```python
from build123d import *

# Parameters (mm, degrees)
BOSS_EXTRUDE1_DEPTH = 22.34
SKETCH3_W           = 42.42
SKETCH3_H           = 6
CUT_EXTRUDE1_DEPTH  = 20.34
SKETCH4_W           = 45.42
SKETCH4_H           = 3.5
CUT_EXTRUDE2_DEPTH  = 20.34
SKETCH6_R           = 0.6
SKETCH6_R_2         = 0.45
SKETCH6_R_3         = 2.25
BOSS_EXTRUDE2_DEPTH = 4
BOSS_EXTRUDE3_START = 2
SKETCH7_R           = 2.25
SKETCH7_R_2         = 1.9
BOSS_EXTRUDE3_DEPTH = 0.5
SKETCH8_W           = 42.42
SKETCH8_H           = 1.5
BOSS_EXTRUDE4_DEPTH = 2
BOSS_EXTRUDE5_DEPTH = 1
FILLET1_R           = 0.5


with BuildPart() as part:
    # Sketch1 → Boss-Extrude1 (new body)
    with BuildSketch(Plane(origin=(0, 0, 0), x_dir=(1, 0, 0), z_dir=(0, 1, 0))):
        Polygon((47.42, 0), (47.42, 6), (45.42, 6), (0, 6), (-2, 6), (-2, 0), (0, 0), (45.42, 0), align=None)
    extrude(amount=BOSS_EXTRUDE1_DEPTH)

    # Sketch3 → Cut-Extrude1 (cut)
    with BuildSketch(Plane(origin=(0, 22.34, 0), x_dir=(1, 0, 0), z_dir=(0, 1, 0))):
        with Locations((22.71, 3)):
            Rectangle(SKETCH3_W, SKETCH3_H)
    extrude(amount=-CUT_EXTRUDE1_DEPTH, mode=Mode.SUBTRACT)

    # Sketch4 → Cut-Extrude2 (cut)
    with BuildSketch(Plane(origin=(0, 22.34, 0), x_dir=(1, 0, 0), z_dir=(0, 1, 0))):
        with Locations((22.71, 2.75)):
            Rectangle(SKETCH4_W, SKETCH4_H)
    extrude(amount=-CUT_EXTRUDE2_DEPTH, mode=Mode.SUBTRACT)

    # Sketch6 → Boss-Extrude2 (add)
    with BuildSketch(Plane.XZ):
        with BuildLine():
            Line((12.71, -6), (19.146099522, -16))
            Line((19.146099522, -16), (19.146099522, -36))
            ThreePointArc((19.146099522, -36), (22.71, -39.563900478), (26.273900478, -36))
            Line((26.273900478, -36), (26.273900478, -16))
            Line((26.273900478, -16), (32.71, -6))
            Line((32.71, -6), (12.71, -6))
        make_face()
        with Locations((22.71, -16)):
            Circle(SKETCH6_R, mode=Mode.SUBTRACT)
        with Locations((22.71, -24.75)):
            Circle(SKETCH6_R_2, mode=Mode.SUBTRACT)
        with Locations((22.71, -32.75)):
            Circle(SKETCH6_R_3, mode=Mode.SUBTRACT)
    extrude(amount=-BOSS_EXTRUDE2_DEPTH)

    # Sketch7 → Boss-Extrude3 (add)
    with BuildSketch(Plane(origin=(0, 2, 0), x_dir=(1, 0, 0), z_dir=(0, 1, 0)).offset(BOSS_EXTRUDE3_START)):
        with Locations((22.71, 32.75)):
            Circle(SKETCH7_R)
        with Locations((22.71, 32.75)):
            Circle(SKETCH7_R_2, mode=Mode.SUBTRACT)
    extrude(amount=-BOSS_EXTRUDE3_DEPTH)

    # Sketch8 → Boss-Extrude4 (add)
    with BuildSketch(Plane(origin=(0, 2, 0), x_dir=(1, 0, 0), z_dir=(0, 1, 0))):
        with Locations((22.71, 5.25)):
            Rectangle(SKETCH8_W, SKETCH8_H)
    extrude(amount=BOSS_EXTRUDE4_DEPTH)

    # Sketch11 → Boss-Extrude5 (add)
    with BuildSketch(Plane.XY):
        Polygon((1.5, 4), (3.5, 2), (1.5, 2), align=None)
        Polygon((43.92, 4), (41.92, 2), (43.92, 2), align=None)
    extrude(amount=-BOSS_EXTRUDE5_DEPTH)

    # Fillet1
    fillet1_edges = [part.edges().sort_by_distance(p)[0] for p in [
        (1.5, 4, -5.25),
        (43.92, 4, -5.25),
        (47.42, 22.34, -3),
        (-2, 22.34, -3),
        (1.5, 22.34, -5.25),
        (43.92, 22.34, -0.5),
        (1.5, 22.34, -0.5),
        (43.92, 22.34, -5.25),
        (45.42, 22.34, -2.75),
        (0, 22.34, -2.75),
        (12.71, 2, -6),
        (32.71, 2, -6),
        (-2, 0, -3),
        (47.42, 0, -3),
    ]]
    fillet(fillet1_edges, radius=FILLET1_R)


solid = part.part
```
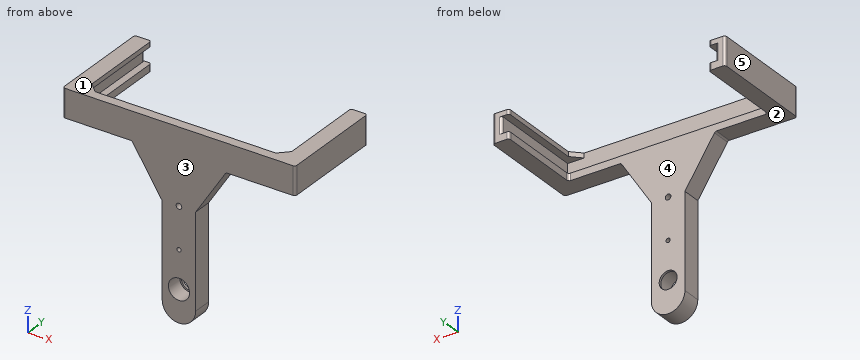
Could you check a few things on this model? Use its own coordinates, in mm. Face numbers are marked on the shaded views. A direction names the side the tool comes from. Round coordinates to 2 decimals unless told otherwise and drop trailing zeros. Loops run counter-clockwise (first coordinate to the right, second up) from the corner with the lowest first, then second, coordinate; pieces in that order, holes last.
Q1. For P1, Ø1.2, axis at x = 1, y = 13.5, coming from the -Z side; P2, Ø5, axis at x = 22.71, z = -32.75, coming from the -Y side; P3, Ø1.5, axis at y = 4.5, z = -15.5, coming from the +X side; P4, Ø1.2, axis at y = 1.5, z = -29.5, coming from the +X side, each with a flat end and sliding along its axis, tell me the tip position at first contact or that it passes through.
Q2. Please list where these lines run through material, in increasing order: L1, parallel to Z at x = 22.71, y = 2.3; L2, parallel to Z at x = 22.71, y = 1.55; L3, parallel to Z at x = 1, y = 12.5.
Q3. Thinking about a two-plate mould opening in X: for the marked faces 3, 4 and 5, which applies, pulls with the +X half, pulls with the -X half, needs draft (parallel to the pull), parting line crosses it, or undercut?
Q4. On a 3-axis mill with a long thin cutter (end or side, diameter ignored), from which of +Z, -Z, +X, -X, +Y, -Y can I reach the whole of each face in a straight line? I mean the marked faces 1 and 2. Say none if no direction works.
Q5. I want a section at B-B (z = -32.75). Write out the boundary of the cut face in (x, y), and give its area (3 significant figures).
Q6. I want a section at A-A (y = 9). Write out the boundary of the cut face in (x, z).
Q7. I want a section at C-C (x = 14). Write out the boundary of the cut face in (y, z).
Q8. I want a section at D-D (z = -27). Write out the boundary of the cut face in (x, y).
Answer below:
1. P1: stops at z = -6
1. P2: stops at y = 0
1. P3: stops at x = 26.96
1. P4: stops at x = 26.27
2. L1: z = -39.56 to -35, -30.5 to -25.2, -24.3 to -16.6, -15.4 to -4.5
2. L2: z = -39.56 to -35, -30.5 to -25.2, -24.3 to -16.6, -15.4 to 0
2. L3: z = -6 to -4.5, -1 to 0
3. face 3: needs draft
3. face 4: undercut
3. face 5: pulls with the -X half
4. face 1: +Z, +X, -X, +Y, -Y
4. face 2: -Z, -X, +Y, -Y
5. outline: (19.15, 0) - (20.46, 0) - (20.46, 3.5) - (20.81, 3.5) - (20.81, 4) - (19.15, 4) - close; (24.61, 3.5) - (24.96, 3.5) - (24.96, 0) - (26.27, 0) - (26.27, 4) - (24.61, 4) - close
5. area: 10.9 mm2
6. outline: (-2, -6) - (1.5, -6) - (1.5, -4.5) - (0, -4.5) - (0, -1) - (1.5, -1) - (1.5, 0) - (-2, 0) - close; (43.92, -6) - (47.42, -6) - (47.42, 0) - (43.92, 0) - (43.92, -1) - (45.42, -1) - (45.42, -4.5) - (43.92, -4.5) - close
7. outline: (0, -8) - (4, -8) - (4, -4.5) - (2, -4.5) - (2, 0) - (0, 0) - close
8. outline: (19.15, 0) - (26.27, 0) - (26.27, 4) - (19.15, 4) - close
